Read the model definition and answer for the solid it produces. Units are mm, in the model's axes. A direction names the side the tool comes from. Coordinates: 2 decimals unless noted, no trailing zeros. Order: outer loops, then holes, each group sorted by start corner. A loop starts at its lowest first (then second) coordinate and runs counter-clockwise, first axis right, second up. Notation, with made-up numbers: (35.25, -8) - (88.25, -8) arc R14 ccw to (88.25, 1) - close; hole circle Ø2 at (-13.75, 40). An arc over 180 degrees is marked (long way). Write item = value, one per line.
from build123d import *

# Parameters (mm, degrees)
ESQUISSE1_W             = 5
ESQUISSE1_H             = 20
BOSS_EXTRU_1_DEPTH      = 21
ESQUISSE2_W             = 25
ESQUISSE2_H             = 20
BOSS_EXTRU_2_DEPTH      = 2
ESQUISSE3_R             = 3.175
BOSS_EXTRU_3_DEPTH      = 7
CONG_1_R                = 10
ESQUISSE5_W             = 5
ESQUISSE5_H             = 20
BOSS_EXTRU_4_DEPTH      = 10
CONG_2_R                = 2
ENL_V_MAT_EXTRU_1_REACH = 37.089
ESQUISSE6_R             = 1.45


with BuildPart() as part:
    # Esquisse1 → Boss.-Extru.1 (new body)
    with BuildSketch(Plane.XY):
        Rectangle(ESQUISSE1_W, ESQUISSE1_H)
    extrude(amount=BOSS_EXTRU_1_DEPTH)

    # Esquisse2 → Boss.-Extru.2 (add)
    with BuildSketch(Plane.XY.offset(21)):
        with Locations((-10, 0)):
            Rectangle(ESQUISSE2_W, ESQUISSE2_H)
    extrude(amount=BOSS_EXTRU_2_DEPTH)

    # Esquisse3 → Boss.-Extru.3 (add)
    with BuildSketch(Plane.XY.offset(23)):
        with Locations((-12.41, 0.35)):
            Circle(ESQUISSE3_R)
    extrude(amount=BOSS_EXTRU_3_DEPTH)

    # Congé1
    cong_1_edges = [part.edges().sort_by_distance(p)[0] for p in [
        (-22.5, 10, 22),
        (-22.5, -10, 22),
    ]]
    fillet(cong_1_edges, radius=CONG_1_R - 0.0001)  # a hair under: the kernel refuses the full size

    # Esquisse5 → Boss.-Extru.4 (add)
    with BuildSketch(Plane(origin=(2.5, 0, 0), x_dir=(0, 0, -1), z_dir=(1, 0, 0))):
        with Locations((-2.5, 0)):
            Rectangle(ESQUISSE5_W, ESQUISSE5_H)
    extrude(amount=BOSS_EXTRU_4_DEPTH)

    # Congé2
    cong_2_edges = [part.edges().sort_by_distance(p)[0] for p in [
        (2.5, 0, 5),
    ]]
    fillet(cong_2_edges, radius=CONG_2_R)

    # Esquisse6 → Enlèv. mat.-Extru.1 (cut, up to next)
    with BuildSketch(Plane.XY.offset(5), mode=Mode.PRIVATE) as enl_v_mat_extru_1_sk1:
        with Locations((8.5, 5)):
            Circle(ESQUISSE6_R)
    enl_v_mat_extru_1_tool1 = extrude(enl_v_mat_extru_1_sk1.sketch, amount=-ENL_V_MAT_EXTRU_1_REACH, mode=Mode.PRIVATE) & part.part
    # Esquisse6 → Enlèv. mat.-Extru.1 (cut, up to next)
    with BuildSketch(Plane.XY.offset(5), mode=Mode.PRIVATE) as enl_v_mat_extru_1_sk2:
        with Locations((8.5, -5)):
            Circle(ESQUISSE6_R)
    enl_v_mat_extru_1_tool2 = extrude(enl_v_mat_extru_1_sk2.sketch, amount=-ENL_V_MAT_EXTRU_1_REACH, mode=Mode.PRIVATE) & part.part
    add(enl_v_mat_extru_1_tool1.solids().sort_by_distance((8.5, 5, 5))[0], mode=Mode.SUBTRACT)
    add(enl_v_mat_extru_1_tool2.solids().sort_by_distance((8.5, -5, 5))[0], mode=Mode.SUBTRACT)


solid = part.part
1) Straight lines are drawn through the part: line 1 along Y through (x, z) = (8.5, 1.1); line 2 along X through (y, z) = (-2.75, 9); line 3 along Z through (x, y) = (-3, 4.5). For each, find the intervals that lie inside material, in ascending order. Write a range as from..to.
Returned:
line_1 = -10..-6.45, -3.55..3.55, 6.45..10
line_2 = -2.5..2.5
line_3 = 21..23
2) The part is cut by section A-A (x = 8.5). Determine the outline of the cut face in (y, z).
Returned:
outline = (-10, 0) - (-6.45, 0) - (-6.45, 5) - (-10, 5) - close; (-3.55, 0) - (3.55, 0) - (3.55, 5) - (-3.55, 5) - close; (6.45, 0) - (10, 0) - (10, 5) - (6.45, 5) - close
3) The part is cut by section C-C (y = 5). Determine the outline of the cut face in (x, z), and give its area (3 significant figures).
Returned:
outline = (-21.16, 21) - (-2.5, 21) - (-2.5, 0) - (7.05, 0) - (7.05, 5) - (4.5, 5) arc R2 cw to (2.5, 7) - (2.5, 23) - (-21.16, 23) - close; (9.95, 0) - (12.5, 0) - (12.5, 5) - (9.95, 5) - close
area = 189 mm^2
4) Determine the mould class of faces 4 (the face through (8, 0, 5)), 5 (the face through (2.5, 0, 15)), 6 (the face through (7.05, -4.94, 2.54)) for opening direction X: pulls with the +X half, pulls with the -X half, needs draft (parallel to the pull), parting line crosses it, or undercut.
Returned:
face_4 = needs draft
face_5 = pulls with the +X half
face_6 = undercut
5) Flat-ended cylindrical pins translate along their axes: pin 1 Ø5 at (x, y) = (-18.5, 0) entering from +Z; pin 2 Ø1.7 at (x, y) = (8.5, 5) entering from +Z; pin 3 Ø5 at (y, z) = (-6, 18) entering from +X; pin 4 Ø6 at (x, y) = (-7, -2.5) entering from -Z. Find the tip coordinate at first contact, or state that the pin passes through.
Returned:
pin_1 = 23
pin_2 = through
pin_3 = 2.5
pin_4 = 21
6) The part is cut by section B-B (z = 4). Determine the outline of the cut face in (x, y), and give its area (3 significant figures).
Returned:
outline = (-2.5, -10) - (12.5, -10) - (12.5, 10) - (-2.5, 10) - close; hole circle Ø2.9 at (8.5, -5); hole circle Ø2.9 at (8.5, 5)
area = 287 mm^2
7) For faces 1 (the face through (-2.5, 0, 10)), 2 (the face through (12.5, 0, 3)), 3 (the face through (-9.38, 1.3, 26.45)), determine the directions among +Z, -Z, +X, -X, +Y, -Y from which every point of the face is accessible in a straight line to the end or side of a thin tool.
Returned:
face_1 = -Z, -X, +Y, -Y
face_2 = +Z, -Z, +X, +Y, -Y
face_3 = +Z
